```python
from build123d import *

# Parameters (mm, degrees)
BOSS_EXTRUDE1_DEPTH     = 1.5
CUT_EXTRUDE4_DEPTH      = 38.286056375
CUT_EXTRUDE4_DEPTH_BACK = 38.286056375
SKETCH4_W               = 0.25
SKETCH4_H               = 3
CUT_EXTRUDE5_DEPTH      = 38.286056375
CUT_EXTRUDE5_DEPTH_BACK = 38.286056375
SKETCH5_R               = 1
FILLET5_R               = 2
BOSS_EXTRUDE2_START     = 2
BOSS_EXTRUDE2_DEPTH     = 2


with BuildPart() as part:
    # Sketch1 → Boss-Extrude1 (new, symmetric)
    with BuildSketch(Plane(origin=(0, 0, 0), x_dir=(1, 0, 0), z_dir=(0, 1, 0))):
        Polygon((-25, -12.5), (25, -12.5), (35, -12.5), (25, 2.5), (24.20625, 2.5), (24.20625, 5.5), (19.20625, 5.5), (19.20625, 12.5), (-19.20625, 12.5), (-19.20625, 5.5), (-24.20625, 5.5), (-24.20625, 2.5), (-25, 2.5), (-35, -12.5), align=None)
    extrude(amount=BOSS_EXTRUDE1_DEPTH, both=True)

    # Sketch4 → Cut-Extrude4 (cut, two sides: drawn at the far end of the back side and taken through both)
    with BuildSketch(Plane(origin=(0, 1.5, 0), x_dir=(1, 0, 0), z_dir=(0, 1, 0)).offset(-CUT_EXTRUDE4_DEPTH_BACK)):
        with Locations((24.08125, 4)):
            Rectangle(SKETCH4_W, SKETCH4_H)
        with Locations((-24.08125, 4)):
            Rectangle(SKETCH4_W, SKETCH4_H)
    extrude(amount=CUT_EXTRUDE4_DEPTH + CUT_EXTRUDE4_DEPTH_BACK, mode=Mode.SUBTRACT)

    # Sketch5 → Cut-Extrude5 (cut, two sides: drawn at the far end of the back side and taken through both)
    with BuildSketch(Plane(origin=(0, 1.5, 0), x_dir=(1, 0, 0), z_dir=(0, 1, 0)).offset(-CUT_EXTRUDE5_DEPTH_BACK)):
        with Locations((-24.663356781, 3.207106781)):
            Circle(SKETCH5_R)
        with Locations((24.663356781, 3.207106781)):
            Circle(SKETCH5_R)
    extrude(amount=CUT_EXTRUDE5_DEPTH + CUT_EXTRUDE5_DEPTH_BACK, mode=Mode.SUBTRACT)

    # Fillet5
    fillet5_edges = [part.edges().sort_by_distance(p)[0] for p in [
        (-35, 0, 12.5),
        (-19.20625, 0, -5.5),
        (19.20625, 0, -5.5),
        (35, 0, 12.5),
    ]]
    fillet(fillet5_edges, radius=FILLET5_R)

    # Sketch6 → Boss-Extrude2 (add)
    with BuildSketch(Plane(origin=(0, 1.5, 0), x_dir=(1, 0, 0), z_dir=(0, 1, 0)).offset(BOSS_EXTRUDE2_START)):
        with BuildLine():
            Line((-24.053996179, 4), (-7.5, 4))
            Line((-7.5, 4), (-7.5, 1))
            Line((-7.5, 1), (-26, 1))
            Line((-26, 1), (-25.121262614, 2.318106079))
            ThreePointArc((-25.121262614, 2.318106079), (-23.819007075, 2.671314309), (-24.053996179, 4))
        make_face()
        with BuildLine():
            Line((26, 1), (25.121262614, 2.318106079))
            ThreePointArc((25.121262614, 2.318106079), (23.819007075, 2.671314309), (24.053996179, 4))
            Line((24.053996179, 4), (7.5, 4))
            Line((7.5, 4), (7.5, 1))
            Line((7.5, 1), (26, 1))
        make_face()
    extrude(amount=-BOSS_EXTRUDE2_DEPTH)


solid = part.part
```
Work out the finished part from the listing and answer in its coordinate system (mm). A direction names the side the tool comes from. Give positions to 0.01 mm unless a question says otherwise; leave off trailing zeros. Loops run counter-clockwise (first coordinate to the right, second up) from the corner with the lowest first, then second, coordinate; pieces in that order, holes last. Notation, with made-up numbers: (-33.5, 80.25) -> (-5.5, 80.25) arc R32 cw to (-5.5, 117.25) -> close; hole circle Ø4 at (-23, 55.5). An arc over 180 degrees is marked (long way). One line per question, with ' | ' between items. Start each with the question number.
1) Section A-A, the plane y = 2.15 is taken. Determine the outline of the cut face in (x, z).
2) Straight lines are drawn through the part: L1, parallel to Y at x = 16.5, z = 9; L2, parallel to Z at x = 18, y = 2.75; L3, parallel to X at y = -0.55, z = -9. For each, find the intervals that lie inside material, in ascending order.
3) Section D-D, the plane x = 14 is taken. Determine the outline of the cut face in (y, z), then the cut area to 3 significant figures.
4) Section C-C, the plane z = -9.75 is taken. Determine the outline of the cut face in (x, y).
5) Each of these flat-tipped pins is pushed along its axis until it touches: pin 1 (1.5 mm diameter, centred on y = 0, z = -10, fed in from -X); pin 2 (12.5 mm diameter, centred on x = -13, z = 0, fed in from +Y); pin 3 (1 mm diameter, centred on y = 2.5, z = -2, fed in from -X); pin 4 (1.7 mm diameter, centred on y = 0.5, z = -4.5, fed in from -X). Where does it stop, or does it pass through?
6) For faces 4 (the face through (19.206, 0, -10)), 5 (the face through (-23, 0, -5.5)), 6 (the face through (-16, 3, -4)), 7 (the face through (-17, 3, -1)), determine the directions among +Z, -Z, +X, -X, +Y, -Y from which every point of the face is accessible in a straight line to the end or side of a thin tool.
7) Section B-B, the plane x = -22 is taken. Determine the outline of the cut face in (y, z), then the cut area to 3 significant figures.
8) Determine the mould class of faces 1 (the face through (23, 0, -5.5)), 2 (the face through (-7.5, 3, -3)), 3 (the face through (19.78, 0.02, -6.1)) for opening direction X: +X half, -X half, draft (parallel to the pull), parting line (faces both ways), or undercut.
Resolved:
1) outline: (-26, -1) -> (-25.12, -2.32) arc R1 cw to (-24.05, -4) -> (-7.5, -4) -> (-7.5, -1) -> close; (7.5, -4) -> (24.05, -4) arc R1 cw to (25.12, -2.32) -> (26, -1) -> (7.5, -1) -> close
2) L1: -1.5 to 1.5 | L2: -4 to -1 | L3: -19.21 to 19.21
3) outline: (-1.5, -12.5) -> (1.5, -12.5) -> (1.5, -4) -> (3.5, -4) -> (3.5, -1) -> (1.5, -1) -> (1.5, 12.5) -> (-1.5, 12.5) -> close | area: 81.0 mm2
4) outline: (-19.21, -1.5) -> (19.21, -1.5) -> (19.21, 1.5) -> (-19.21, 1.5) -> close
5) pin 1: x = -19.21 | pin 2: y = 3.5 | pin 3: x = -25.67 | pin 4: x = -23.96
6) face 4: -Z, +X, +Y, -Y | face 5: -Z, -X, +Y, -Y | face 6: -Z, +X, -X, +Y | face 7: +Z, +X, -X, +Y
7) outline: (-1.5, -5.5) -> (1.5, -5.5) -> (1.5, -4) -> (3.5, -4) -> (3.5, -1) -> (1.5, -1) -> (1.5, 12.5) -> (-1.5, 12.5) -> close | area: 60.0 mm2
8) face 1: draft | face 2: undercut | face 3: +X half
